Check sheet for the modelled part. Datum: model origin and axes. Units: mm. A direction names the side the tool comes from. Give positions to 0.01 mm unless a question says otherwise; leave off trailing zeros. Loops run counter-clockwise (first coordinate to the right, second up) from the corner with the lowest first, then second, coordinate; pieces in that order, holes last. Notation, with made-up numbers: (83.5, -11) - (103.5, -11) arc R23 ccw to (103.5, 1) - close; hole circle Ø3 at (-30.75, -20). An arc over 180 degrees is marked (long way). Answer in a Markdown table with one row per item. Add a question column.
(1) Thickness scan on L1, parallel to Z at x = 16.25, y = 3.5; L2, parallel to X at y = -11.75, z = 0.2; L3, parallel to X at y = -7.25, z = 2.35. Record the ranges inside material, lowest first.
(2) Sectioned sample at C-C on x = 3. Enter the section's corners in (y, z), then the cut area to 3 significant figures.
(3) Sectioned sample at D-D on y = -14. Enter the section's corners in (x, z), then the cut area to 3 significant figures.
(4) Go/stop test with a flat-tipped pin: P1, Ø0.6, axis at y = -9, z = 0.5, coming from the +X side. Record where the tip stops, or that it passes through.
(5) Set-up check for faces 1 (the face through (6.68, -9.74, 2.25)), 2 (the face through (6.72, -5.24, 2.25)), 3 (the face through (17, 0, 1)), 4 (the face through (0, -8, 1)), 5 (the face through (9.32, -5.26, 2.25)): record each of +Z, -Z, +X, -X, +Y, -Y from which the full face is reachable in a straight line by a thin tool's end or side.
(6) Sectioned sample at A-A on z = 1.6. Enter the section's corners in (x, y), then the cut area to 3 significant figures.
(7) Sectioned sample at B-B on y = -6.75. Enter the section's corners in (x, z), then the cut area to 3 significant figures.
from build123d import *

# Parameters (mm, degrees)
CROQUIS1_W              = 16
CROQUIS1_H              = 15
SALIENTE_EXTRUIR3_DEPTH = 2
REDONDEO1_R             = 2
SALIENTE_EXTRUIR4_DEPTH = 1
REDONDEO2_R             = 0.5


with BuildPart() as part:
    # Croquis1 → Saliente-Extruir3 (new body)
    with BuildSketch(Plane.XY):
        Polygon((-1.5, 0), (0, 0), (16, 0), (17.5, 0), (17.5, 5), (-1.5, 5), align=None)
        with Locations((8, -7.5)):
            Rectangle(CROQUIS1_W, CROQUIS1_H)
    extrude(amount=SALIENTE_EXTRUIR3_DEPTH)

    # Redondeo1
    redondeo1_edges = [part.edges().sort_by_distance(p)[0] for p in [
        (-1.5, 5, 1),
        (17.5, 5, 1),
    ]]
    fillet(redondeo1_edges, radius=REDONDEO1_R)

    # Croquis3 → Saliente-Extruir4 (add)
    with BuildSketch(Plane.XY.offset(2)):
        Polygon((8, -4.5), (5.401923789, -6), (5.401923789, -9), (8, -10.5), (10.598076211, -9), (10.598076211, -6), align=None)
    extrude(amount=SALIENTE_EXTRUIR4_DEPTH)

    # Redondeo2
    redondeo2_edges = [part.edges().sort_by_distance(p)[0] for p in [
        (9.299038106, -5.25, 3),
        (6.700961894, -5.25, 3),
        (5.401923789, -7.5, 3),
        (6.700961894, -9.75, 3),
        (9.299038106, -9.75, 3),
        (10.598076211, -7.5, 3),
    ]]
    fillet(redondeo2_edges, radius=REDONDEO2_R)


solid = part.part
Reply:
| question | item | result |
|---|---|---|
| 1 | L1 | 0 to 2 |
| 1 | L2 | 0 to 16 |
| 1 | L3 | 5.4 to 10.6 |
| 2 | outline | (-15, 0) - (5, 0) - (5, 2) - (-15, 2) - close |
| 2 | area | 40.0 mm^2 |
| 3 | outline | (0, 0) - (16, 0) - (16, 2) - (0, 2) - close |
| 3 | area | 32.0 mm^2 |
| 4 | P1 | x = 16 |
| 5 | face 1 | +Z, -X, -Y |
| 5 | face 2 | +Z, -X, +Y |
| 5 | face 3 | +Z, -Z, +X, -Y |
| 5 | face 4 | +Z, -Z, -X, -Y |
| 5 | face 5 | +Z, +X, +Y |
| 6 | outline | (-1.5, 0) - (0, 0) - (0, -15) - (16, -15) - (16, 0) - (17.5, 0) - (17.5, 3) arc R2 ccw to (15.5, 5) - (0.5, 5) arc R2 ccw to (-1.5, 3) - close |
| 6 | area | 333 mm^2 |
| 7 | outline | (0, 0) - (16, 0) - (16, 2) - (10.6, 2) - (10.6, 2.5) arc R0.5 ccw to (10.1, 3) - (5.9, 3) arc R0.5 ccw to (5.4, 2.5) - (5.4, 2) - (0, 2) - close |
| 7 | area | 37.1 mm^2 |
